```python
from build123d import *

# Parameters (mm, degrees)
SKETCH1_W               = 650
SKETCH1_H               = 650
BOSS_EXTRUDE1_DEPTH     = 8
BOSS_EXTRUDE2_DEPTH     = 650
CUT_EXTRUDE2_DEPTH      = 921.277302922
CUT_EXTRUDE2_DEPTH_BACK = 921.277302922
SKETCH4_R               = 16.05
CUT_EXTRUDE1_DEPTH      = 920.932062709
CUT_EXTRUDE1_DEPTH_BACK = 920.932062709
SKETCH2_R               = 210
CUT_EXTRUDE3_DEPTH      = 921.277302998
CUT_EXTRUDE3_DEPTH_BACK = 110
CUT_EXTRUDE4_DEPTH      = 110
CUT_EXTRUDE5_DEPTH      = 920.932062713
CUT_EXTRUDE5_DEPTH_BACK = 920.932062713
SKETCH7_OUTSIDE_W       = 836.056
SKETCH7_OUTSIDE_H       = 836.056
SKETCH7_OUTSIDE_W_2     = 260
SKETCH7_OUTSIDE_H_2     = 231.544504505
BOSS_EXTRUDE3_DEPTH     = 170
SKETCH9_W               = 9.9
SKETCH9_H               = 4
BOSS_EXTRUDE4_DEPTH     = 170
CUT_EXTRUDE6_DEPTH      = 800.941879143
CUT_EXTRUDE6_DEPTH_BACK = 800.941879143
SKETCH10_R              = 210
SKETCH11_W              = 50
SKETCH11_H              = 3
BOSS_EXTRUDE5_DEPTH     = 100
CUT_EXTRUDE7_DEPTH      = 800.81358281
CUT_EXTRUDE7_DEPTH_BACK = 800.81358281
SKETCH12_R              = 1.75
CUT_EXTRUDE8_DEPTH      = 706.164040729
CUT_EXTRUDE8_DEPTH_BACK = 10
SKETCH13_R              = 2.75
CUT_EXTRUDE9_START      = -10
SKETCH14_R              = 2.75
CUT_EXTRUDE9_DEPTH      = 10
CUT_EXTRUDE10_DEPTH     = 3
LPATTERN1_COUNT         = 3
LPATTERN1_PITCH         = 40
CUT_EXTRUDE11_DEPTH     = 3
LPATTERN2_COUNT         = 3
LPATTERN2_PITCH         = 40
SKETCH17_W              = 15.1
SKETCH17_H              = 100.1
CUT_EXTRUDE12_DEPTH     = 3


with BuildPart() as part:
    # Sketch1 → Boss-Extrude1 (new body)
    with BuildSketch(Plane(origin=(0, 0, 0), x_dir=(1, 0, 0), z_dir=(0, 1, 0))):
        with Locations((325, 325)):
            Rectangle(SKETCH1_W, SKETCH1_H)
    extrude(amount=BOSS_EXTRUDE1_DEPTH)

    # Sketch3 → Boss-Extrude2 (add)
    with BuildSketch(Plane.XY):
        Polygon((300, 43.707142143), (350, 43.707142143), (385, 8), (265, 8), align=None)
    extrude(amount=-BOSS_EXTRUDE2_DEPTH)

    # Sketch4 → Cut-Extrude2 (cut, two sides: drawn at the far end of the back side and taken through both)
    with BuildSketch(Plane.XY.offset(-CUT_EXTRUDE2_DEPTH_BACK)):
        with Locations((325, 25)):
            Circle(SKETCH4_R)
    extrude(amount=CUT_EXTRUDE2_DEPTH + CUT_EXTRUDE2_DEPTH_BACK, mode=Mode.SUBTRACT)

    # Sketch2 → Cut-Extrude1 (cut, two sides: drawn at the far end of the back side and taken through both)
    with BuildSketch(Plane(origin=(0, 8, 0), x_dir=(1, 0, 0), z_dir=(0, 1, 0)).offset(-CUT_EXTRUDE1_DEPTH_BACK)):
        with Locations(Location((325, 325, 0), (0, 0, 270))):
            Circle(SKETCH2_R)
    extrude(amount=CUT_EXTRUDE1_DEPTH + CUT_EXTRUDE1_DEPTH_BACK, mode=Mode.SUBTRACT)

    # Sketch5 → Cut-Extrude3 (cut, two sides: drawn at the far end of the back side and taken through both)
    with BuildSketch(Plane.XY.offset(-CUT_EXTRUDE3_DEPTH_BACK)):
        Polygon((300, 43.707142143), (350, 43.707142143), (365.396078824, 28), (350, 28), (350, 8), (300, 8), (300, 28), (284.603921176, 28), align=None)
    extrude(amount=CUT_EXTRUDE3_DEPTH + CUT_EXTRUDE3_DEPTH_BACK, mode=Mode.SUBTRACT)

    # Sketch6 → Cut-Extrude4 (cut)
    with BuildSketch(Plane(origin=(0, 0, -650), x_dir=(-1, 0, 0), z_dir=(0, 0, -1))):
        Polygon((-350, 43.707142143), (-300, 43.707142143), (-284.603921176, 28), (-300, 28), (-300, 8), (-350, 8), (-350, 28), (-365.396078824, 28), align=None)
    extrude(amount=-CUT_EXTRUDE4_DEPTH, mode=Mode.SUBTRACT)

    # Sketch7 outside → Cut-Extrude5 (cut, two sides: drawn at the far end of the back side and taken through both)
    with BuildSketch(Plane(origin=(0, 8, 0), x_dir=(1, 0, 0), z_dir=(0, 1, 0)).offset(-CUT_EXTRUDE5_DEPTH_BACK)):
        with Locations((325, 325)):
            Rectangle(SKETCH7_OUTSIDE_W, SKETCH7_OUTSIDE_H)
        with Locations((325, 570.772252253)):
            Rectangle(SKETCH7_OUTSIDE_W_2, SKETCH7_OUTSIDE_H_2, mode=Mode.SUBTRACT)
    extrude(amount=CUT_EXTRUDE5_DEPTH + CUT_EXTRUDE5_DEPTH_BACK, mode=Mode.SUBTRACT)

    # Sketch8 → Boss-Extrude3 (add)
    with BuildSketch(Plane(origin=(0, 0, -650), x_dir=(-1, 0, 0), z_dir=(0, 0, -1))):
        Polygon((-455, 8), (-455, 28), (-445, 28), (-445, 17), (-435.61916848, 8), align=None)
        Polygon((-195, 8), (-195, 28), (-205, 28), (-205, 17), (-214.38083152, 8), align=None)
    extrude(amount=-BOSS_EXTRUDE3_DEPTH)

    # Sketch9 → Boss-Extrude4 (add)
    with BuildSketch(Plane(origin=(0, 0, -650), x_dir=(-1, 0, 0), z_dir=(0, 0, -1))):
        with Locations((-459.95, 5)):
            Rectangle(SKETCH9_W, SKETCH9_H)
        with Locations((-190.05, 5)):
            Rectangle(SKETCH9_W, SKETCH9_H)
    extrude(amount=-BOSS_EXTRUDE4_DEPTH)

    # Sketch10 → Cut-Extrude6 (cut, two sides: drawn at the far end of the back side and taken through both)
    with BuildSketch(Plane(origin=(0, 8, 0), x_dir=(1, 0, 0), z_dir=(0, 1, 0)).offset(-CUT_EXTRUDE6_DEPTH_BACK)):
        with Locations((325, 325)):
            Circle(SKETCH10_R)
    extrude(amount=CUT_EXTRUDE6_DEPTH + CUT_EXTRUDE6_DEPTH_BACK, mode=Mode.SUBTRACT)

    # Sketch11 → Boss-Extrude5 (add)
    with BuildSketch(Plane(origin=(0, 0, -650), x_dir=(-1, 0, 0), z_dir=(0, 0, -1))):
        with Locations((-325, 9.5)):
            Rectangle(SKETCH11_W, SKETCH11_H)
    extrude(amount=-BOSS_EXTRUDE5_DEPTH)

    # Sketch12 → Cut-Extrude7 (cut, two sides: drawn at the far end of the back side and taken through both)
    with BuildSketch(Plane(origin=(0, 11, 0), x_dir=(1, 0, 0), z_dir=(0, 1, 0)).offset(-CUT_EXTRUDE7_DEPTH_BACK)):
        with Locations(Location((305.5, 640.7, 0), (0, 0, 270))):
            Circle(SKETCH12_R)
        with Locations(Location((344.5, 640.7, 0), (0, 0, 270))):
            Circle(SKETCH12_R)
        with Locations(Location((344.5, 602.7, 0), (0, 0, 270))):
            Circle(SKETCH12_R)
        with Locations(Location((305.5, 602.7, 0), (0, 0, 270))):
            Circle(SKETCH12_R)
    extrude(amount=CUT_EXTRUDE7_DEPTH + CUT_EXTRUDE7_DEPTH_BACK, mode=Mode.SUBTRACT)

    # Sketch13 → Cut-Extrude8 (cut, two sides: drawn at the far end of the back side and taken through both)
    with BuildSketch(Plane(origin=(455, 0, 0), x_dir=(0, 0, -1), z_dir=(1, 0, 0)).offset(-CUT_EXTRUDE8_DEPTH_BACK)):
        with Locations((610, 23)):
            Circle(SKETCH13_R)
        with Locations((570, 23)):
            Circle(SKETCH13_R)
        with Locations((530, 23)):
            Circle(SKETCH13_R)
    extrude(amount=CUT_EXTRUDE8_DEPTH + CUT_EXTRUDE8_DEPTH_BACK, mode=Mode.SUBTRACT)

    # Sketch14 → Cut-Extrude9 (cut)
    with BuildSketch(Plane.ZY.offset(-195).offset(CUT_EXTRUDE9_START)):
        with Locations(Location((-610, 23, 0), (0, 0, 180))):
            Circle(SKETCH14_R)
        with Locations(Location((-570, 23, 0), (0, 0, 180))):
            Circle(SKETCH14_R)
        with Locations(Location((-530, 23, 0), (0, 0, 180))):
            Circle(SKETCH14_R)
    extrude(amount=CUT_EXTRUDE9_DEPTH, mode=Mode.SUBTRACT)

    # Sketch15 → Cut-Extrude10 (cut)
    with BuildSketch(Plane(origin=(205, 0, 0), x_dir=(0, 0, -1), z_dir=(1, 0, 0))):
        Polygon((530, 27.1), (527.63, 27.1), (525.262863896, 23), (527.63, 18.9), (530, 18.9), (532.37, 18.9), (534.737136104, 23), (532.37, 27.1), align=None)
    cut_extrude10 = extrude(amount=-CUT_EXTRUDE10_DEPTH, mode=Mode.SUBTRACT)

    # LPattern1: Cut-Extrude10 ×3
    with Locations(*[(0, 0, -i * LPATTERN1_PITCH) for i in range(1, LPATTERN1_COUNT)]):
        add(cut_extrude10, mode=Mode.SUBTRACT)

    # Sketch16 → Cut-Extrude11 (cut)
    with BuildSketch(Plane.ZY.offset(-445)):
        Polygon((-610, 27.1), (-607.63, 27.1), (-605.262863896, 23), (-607.63, 18.9), (-610, 18.9), (-612.37, 18.9), (-614.737136104, 23), (-612.37, 27.1), align=None)
    cut_extrude11 = extrude(amount=-CUT_EXTRUDE11_DEPTH, mode=Mode.SUBTRACT)

    # LPattern2: Cut-Extrude11 ×3
    with Locations(*[(0, 0, i * LPATTERN2_PITCH) for i in range(1, LPATTERN2_COUNT)]):
        add(cut_extrude11, mode=Mode.SUBTRACT)

    # Sketch17 → Cut-Extrude12 (cut)
    with BuildSketch(Plane(origin=(0, 0, 0), x_dir=(-1, 0, 0), z_dir=(0, -1, 0))):
        with Locations((-325.05, 589.95)):
            Rectangle(SKETCH17_W, SKETCH17_H)
    extrude(amount=-CUT_EXTRUDE12_DEPTH, mode=Mode.SUBTRACT)


solid = part.part
```
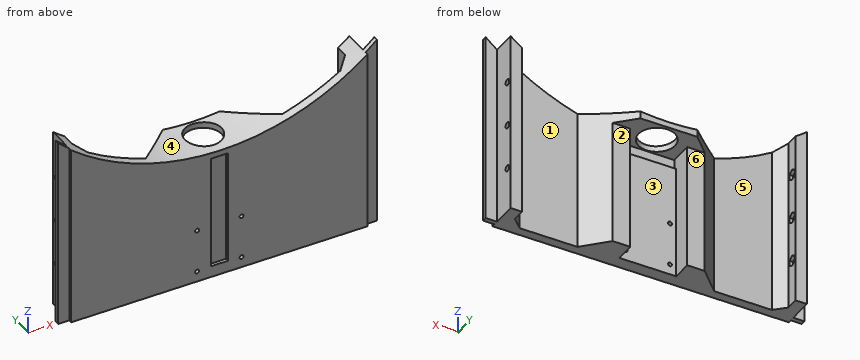
The listing builds one solid part. Answer for the finished solid, in the listing's coordinates (mm). Face numbers are marked on the shaded views. A direction names the side the tool comes from. Coordinates: 2 decimals unless noted, no trailing zeros. Loops run counter-clockwise (first coordinate to the right, second up) from the corner with the lowest first, then second, coordinate; pieces in that order, holes last. Notation, with made-up numbers: (69.25, 74) -> (94.25, 74) arc R36 cw to (94.25, 108) -> close; hole circle Ø10 at (-34, 22). An arc over 180 degrees is marked (long way). Use one line per item in the form item = value. Start each with the question number.
Item 1: The part is cut by section D-D on x = 417.5. Determine the outline of the cut face in (y, z), then the cut area to 3 significant figures.
Item 2: Flat-ended cylindrical pins translate along their axes: pin 1 Ø5 at (x, y) = (358, 18.5) entering from +Z; pin 2 Ø0.9 at (y, z) = (1, -580) entering from -X; pin 3 Ø0.9 at (x, z) = (203.5, -529) entering from +Y. Find the tip coordinate at first contact, or state that the pin passes through.
Item 3: Consider L1, parallel to X at y = 3.5, z = -640.7; L2, parallel to Y at x = 450, z = -570; L3, parallel to Z at x = 451.75, y = 23. Determine where each line is inside the solid, lowest interval first. Write a range as [from, to].
Item 4: A tool of negligible diameter and unlimited length cuts with its end or side. For the marked faces 3, 4, 5 and 6, from which of +Z, -Z, +X, -X, +Y, -Y can it reach the whole face along a straight path? Write none if from no direction.
Item 5: The part is cut by section C-C on y = 31. Determine the outline of the cut face in (x, z), then the cut area to 3 significant figures.
Item 6: The part is cut by section A-A on x = 325. Determine the outline of the cut face in (y, z).
Item 7: The mould has two halves that part along X. Classify the marked faces 1 and 2: released by +X, released by -X, zero draft, split by the parting line, or undercut.
Answer key:
q1.outline = (0, -650) -> (8, -650) -> (8, -513.53) -> (0, -513.53) -> close
q1.area = 1,090 mm2
q2.pin_1 = -531.98
q2.pin_2 = 195
q2.pin_3 = 28
q3.L1 = [185.1, 303.75], [307.25, 342.75], [346.25, 464.9]
q3.L2 = [0, 20.25], [25.75, 28]
q3.L3 = [-650, -612.75], [-607.25, -572.75], [-567.25, -532.75], [-527.25, -492.43]
q4.face_3 = -Z, +Y
q4.face_4 = +Z, +Y, -Y
q4.face_5 = +Z, -Z, +Y
q4.face_6 = -Z, +X, -X, +Y
q5.outline = (287.54, -540) -> (310.11, -540) -> (310.11, -534.47) arc R210 cw to (287.54, -531.63) -> close; (339.89, -540) -> (362.46, -540) -> (362.46, -531.63) arc R210 cw to (339.89, -534.47) -> close
q5.area = 304 mm2
q6.outline = (0, -650) -> (11, -650) -> (11, -550) -> (8, -550) -> (8, -540) -> (8.95, -540) -> (8.95, -535) -> (0, -535) -> (0, -539.9) -> (3, -539.9) -> (3, -640) -> (0, -640) -> close; (41.05, -540) -> (43.71, -540) -> (43.71, -535) -> (41.05, -535) -> close
q7.face_1 = undercut
q7.face_2 = zero draft
